Could you check a few things on this drawing? It's one solid part, dimensions in mm from its lowest x, y, z. Round coordinates to 2 decimals unless told otherwise and drop trailing zeros. Use a Markdown table: item, result. Add a question column.
(1) I'm going to push flat-ended pins straight in: P1, Ø10, axis at x = 83, z = 20, coming from the +Y side; P2, Ø8, axis at x = 72, z = 28, coming from the +Y side; P3, Ø1.5, axis at x = 92, z = 13.5, coming from the -Y side; P4, Ø15, axis at x = 53.975, y = 53.975, coming from the -Z side. Where does each tip first touch, or does it pass through?
(2) If I drill on probe 1 along Y at (x, z) = (53.5, 45); probe 2 along X at (y, z) = (51, 52.5); probe 3 along Y at (x, z) = (55, 8) (1 decimal), over which ranges is the centre line in solid material (lowest first)?
(3) Thinking about a two-plate mould opening in Y: for the marked faces 1, 2 and 3, which applies, pulls with the +Y half, pulls with the -Y half, needs draft (parallel to the pull), parting line crosses it, or undercut?
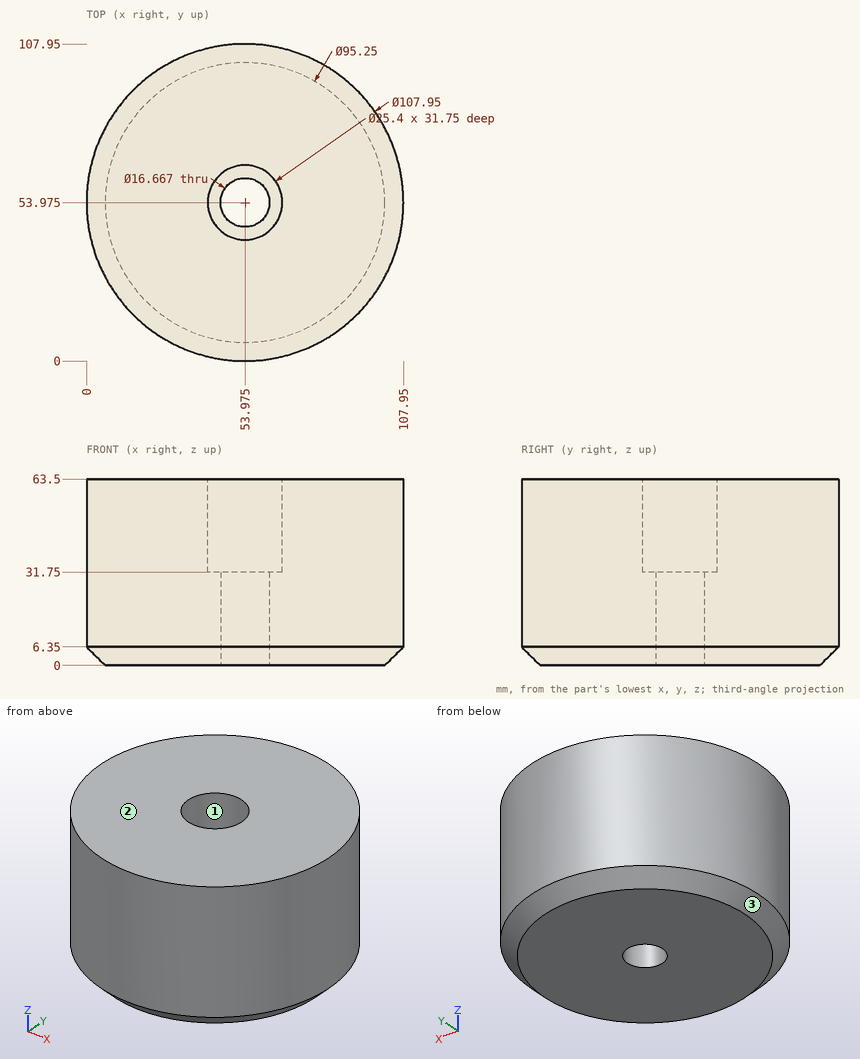
Taken from the geometry:
| question | item | result |
|---|---|---|
| 1 | P1 | stops at y = 102.31 |
| 1 | P2 | stops at y = 106.1 |
| 1 | P3 | stops at y = 14.94 |
| 1 | P4 | passes through |
| 2 | probe 1 | y = 0 to 41.28, 66.67 to 107.95 |
| 2 | probe 2 | x = 0.08 to 41.63, 66.32 to 107.87 |
| 2 | probe 3 | y = 0 to 45.7, 62.2 to 107.9 |
| 3 | face 1 | undercut |
| 3 | face 2 | needs draft |
| 3 | face 3 | parting line crosses it |
